Could you check a few things on this model? Use its own coordinates, in mm. A direction names the side the tool comes from. Round coordinates to 2 decimals unless told otherwise and drop trailing zeros. Write each loop counter-clockwise with the first axis right and the second up, starting at its lowest first coordinate (ties: lowest second). Pieces come first, ordered by that corner, then holes. Notation, with made-up numbers: M 68,32.5 L 121,32.5 A15 cw 121,59.5 Z; hole C -29.75,13.25 d7. An arc over 180 degrees is marked long. One line per question, with ' | ' between items. Start each with the question number.
Autodesk Inventor part; units mm, degrees
ref_plane "YZ Plane" through (0, 0, 0) normal (1, 0, 0) x (0, 1, 0)
ref_plane "XZ Plane" through (0, 0, 0) normal (0, 1, 0) x (-1, 0, 0)
ref_plane "XY Plane" through (0, 0, 0) normal (0, 0, 1) x (1, 0, 0)
sketch "Sketch1" plane through (0, 0, 0) normal (0, 0, 1) x (1, 0, 0)
  circle A0 centre (4, 4) radius 1.2
  circle A1 centre (4, 4) radius 1.5
  point P0 (0, 0)
  dimension "d0" = 3
extrude "Extrusion1" add sketch "Sketch1" against normal blind 10 contours A0 | A1
sketch "Sketch2" plane through (4, 4, 0) normal (0, 0, 1) x (1, 0, 0)
  circle A0 centre (0, 0) radius 1.5
  circle A1 centre (0, 0) radius 2.8
  point P0 (-4, -4)
  dimension "d3" = 5.6
extrude "Extrusion2" add sketch "Sketch2" along normal blind 3 contours A0 | A1
fillet "Fillet1" radius 0.3 1 edges at (1.2, 4, 3)
sketch "Sketch3" plane through (4, 4, 0) normal (0, 0, -1) x (-1, 0, 0)
  circle A0 centre (0, 0) radius 2.8
  circle A1 centre (0, 0) radius 1.5
  circle A2 centre (0, 0) radius 2.75
  point P0 (4, -4)
  dimension "d7" = 5.5
extrude "Extrusion3" cut sketch "Sketch3" against normal blind 0.5 contours A0
sketch "Sketch4" plane through (4, 4, 3) normal (0, 0, 1) x (1, 0, 0)
  circle A0 centre (0, 0) radius 2.5
  line L0 (0.7217, 1.25) -> (1.4434, 0)
  line L1 (1.4434, 0) -> (0.7217, -1.25)
  line L2 (0.7217, -1.25) -> (-0.7217, -1.25)
  line L3 (-0.7217, -1.25) -> (-1.4434, 0)
  line L4 (-1.4434, 0) -> (-0.7217, 1.25)
  line L5 (-0.7217, 1.25) -> (0.7217, 1.25)
  point P0 (-4, -4)
  dimension "d10" = 2.5
extrude "Extrusion4" cut sketch "Sketch4" against normal blind 2 contours L0 L1 L2 L3 L4 L5
thread "Thread1"
properties part number "m3 6" material "Steel"
1. If we mould it in two halves opening along Y, with no side actions, what happens to faces 4 (the face through (4, 2.75, 2)), 5 (the face through (2.73, 1.56, 0.25)), 6 (the face through (5.1, 2.9, 3))? For each: released by +Y, released by -Y, zero draft, split by the parting line, or undercut.
2. Which directions (+Z, -Z, +X, -X, +Y, -Y) give clear straight access to the entire face, cutting with the end or side of a thin tool? Please do faces 1 (the face through (1.936, 2.108, 1.585)), 2 (the face through (2.912, 4.616, 2.014)), 3 (the face through (5.43, 4.45, -4.93)).
3. I'm going to push flat-ended pins straight in: P1, Ø3, axis at y = 2, z = -3.5, coming from the -X side; P2, Ø1, axis at x = 4, y = 4.5, coming from the +Z side. Where does each tip first touch, or does it pass through?
4. Suppose I cut it at B-B (z = -9). Write out the boundary of the cut face in (x, y).
5. I need wall thicknesses on line 1 along Y through (x, z) = (4, -9); line 2 along Z through (x, y) = (3.65, 4.9); line 3 along Y through (x, z) = (4.4, -8.5). Which ranges of each line are inside material? Lowest first, please. Write a range as from..to.
6. Suppose I cut it at A-A (x = 4). Write out the boundary of the cut face in (y, z), and give its area (3 significant figures).
Computed:
1) face 4: undercut | face 5: split by the parting line | face 6: zero draft
2) face 1: +Z, -Z | face 2: +Z | face 3: -Z
3) P1: stops at x = 2.59 | P2: stops at z = 1
4) outline: C 4,4 d3
5) line 1: y = 2.5..5.5 | line 2: z = -10..1 | line 3: y = 2.55..5.45
6) outline: M 1.2,0.5 L 1.25,0.5 L 1.25,0 L 2.5,0 L 2.5,-10 L 5.5,-10 L 5.5,0 L 6.75,0 L 6.75,0.5 L 6.8,0.5 L 6.8,2.7 A0.3 ccw 6.5,3 L 5.25,3 L 5.25,1 L 2.75,1 L 2.75,3 L 1.5,3 A0.3 ccw 1.2,2.7 Z | area: 41.7 mm²
